from build123d import *

# Parameters (mm, degrees)
F0_W     = 100
F0_H     = 100
F0_W_2   = 90
F0_H_2   = 90
F1_DEPTH = 100
F2_R     = 15
F3_DEPTH = 10
F4_R     = 15
F5_DEPTH = 25


with BuildPart() as f1:
    # F0 (on Top) → F1 (new body)
    with BuildSketch(Plane.XY):
        Rectangle(F0_W, F0_H)
        Rectangle(F0_W_2, F0_H_2, mode=Mode.SUBTRACT)
    extrude(amount=F1_DEPTH)

    # F2 (on face) → F3 (cut)
    with BuildSketch(Plane.XZ.offset(50)):
        with Locations((-4.887418, 68.32698)):
            Circle(F2_R)
    extrude(amount=F3_DEPTH, mode=Mode.SUBTRACT)

    # F4 (on face) → F5 (cut)
    with BuildSketch(Plane.XZ.offset(50)):
        with Locations((-4.508148, 66.540122)):
            Circle(F4_R)
    extrude(amount=-F5_DEPTH, mode=Mode.SUBTRACT)


solid = f1.part
For this review, take the finished solid that the model builds, in its own axes (mm). A direction names the side the tool comes from. Coordinates: 2 decimals unless noted, no trailing zeros. Order: outer loops, then holes, each group sorted by start corner. A loop starts at its lowest first (then second) coordinate and runs counter-clockwise, first axis right, second up. Notation, with made-up numbers: (10, 57.5) -> (66, 57.5) arc R21 cw to (66, 78.5) -> close; hole circle Ø1 at (-2, 37.25). An arc over 180 degrees is marked (long way). Return JSON: item names as keys, results as strings.
1. For line 1 (X direction, y = -27, z = 86); line 2 (Y direction, x = -13.5, z = 59.5), list the stretches that pass through material, from the lowest coordinate up. Write a range as from..to.
Answer block:
{"line 1": "-50..-45, 45..50", "line 2": "45..50"}
2. For pin 1 Ø18 at (x, z) = (-4.51, 66.54) entering from -Y, flat-tipped, find the tip position at first contact; note if it passes through.
Answer block:
{"pin 1": "y = 45"}
3. We need section B-B on x = 33.5. Write out the cut boundary in (y, z).
Answer block:
{"outline": "(-50, 0) -> (-45, 0) -> (-45, 100) -> (-50, 100) -> close; (45, 0) -> (50, 0) -> (50, 100) -> (45, 100) -> close"}
4. We need section D-D on x = -10. Write out the cut boundary in (y, z), and give its area (3 significant figures).
Answer block:
{"outline": "(-50, 0) -> (-45, 0) -> (-45, 52.58) -> (-50, 52.58) -> close; (-50, 80.5) -> (-45, 80.5) -> (-45, 100) -> (-50, 100) -> close; (45, 0) -> (50, 0) -> (50, 100) -> (45, 100) -> close", "area": "860 mm²"}
5. We need section A-A on z = 49. Write out the cut boundary in (x, y).
Answer block:
{"outline": "(-50, -50) -> (50, -50) -> (50, 50) -> (-50, 50) -> close; hole (-45, -45) -> (45, -45) -> (45, 45) -> (-45, 45) -> close"}
6. Machinability: for faces 4 (the flat face through (-1, 50, 49)), 5 (the cylindrical face through (-7.76, -47.535, 51.897)), 6 (the flat face through (-1, 45, 49)), which of the approach directions +Z, -Z, +X, -X, +Y, -Y give a long, thin tool a straight path to every point of the face, cutting with its end or side? Answer none if there is none.
Answer block:
{"face 4": "+Z, -Z, +X, -X, +Y", "face 5": "-Y", "face 6": "+Z, -Z"}
7. The part is to be moulded in two halves that separate along X. For faces 1 (the flat face through (-50, -1, 49)), 2 (the flat face through (-4, -48, 100)), 3 (the flat face through (-45, -1, 49)), say which applies: +X half, -X half, draft (parallel to the pull), parting line (faces both ways), or undercut.
Answer block:
{"face 1": "-X half", "face 2": "draft", "face 3": "undercut"}
